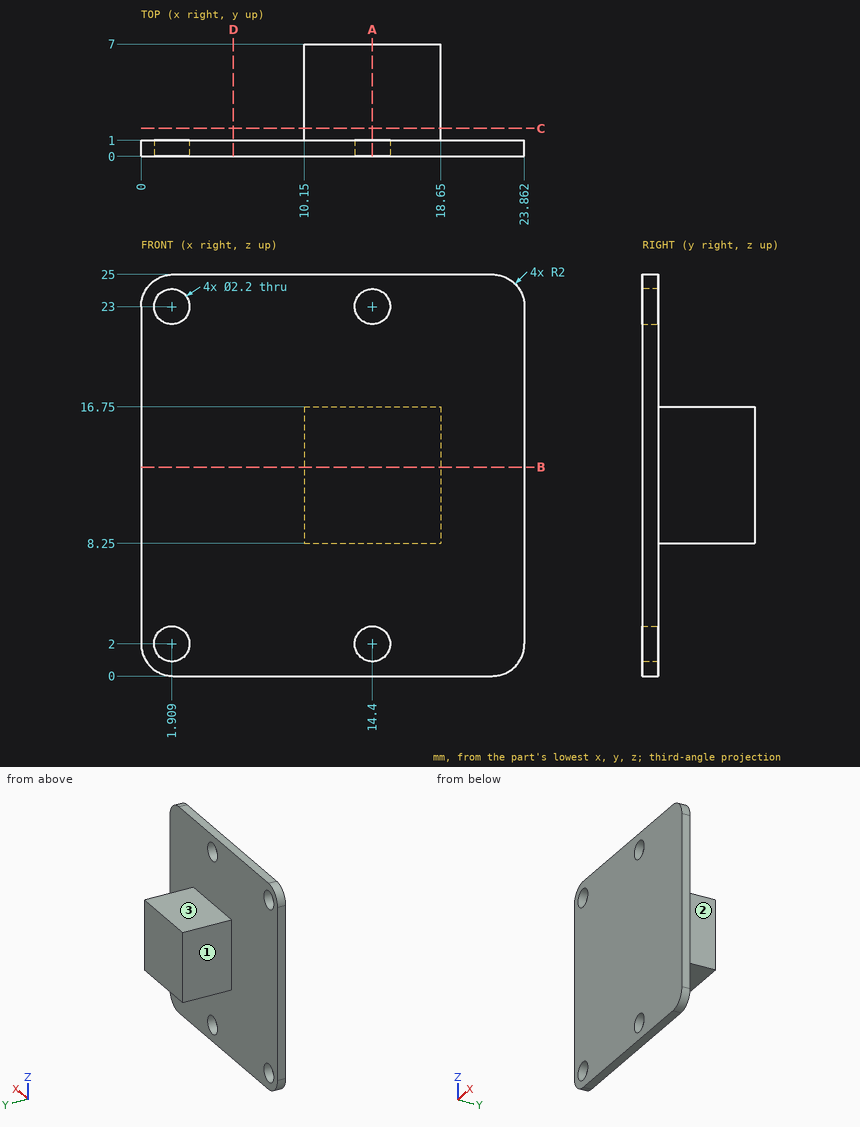
The figure shows three views and two pictorial views of one solid part (mm, origin at its lowest corner). Answer the questions. A direction names the side the tool comes from. Round coordinates to 2 decimals unless told otherwise and drop trailing zeros. Order: outer loops, then holes, each group sorted by start corner. A loop starts at its lowest first (then second) coordinate and runs counter-clockwise, first axis right, second up. Notation, with made-up numbers: M -6.75,85 L 25.25,85 A14 ccw 25.25,103 Z; hole C 40,2.5 d1. An arc over 180 degrees is marked long. Answer in a Markdown table with one row per item. Add a question column.
1) Which of the six approach directions +Z, -Z, +X, -X, +Y, -Y give full straight-line access (tool end or side, diameter ignored) to the marked faces 1, 2 and 3?
2) The part is cut by section B-B on z = 13. Determine the outline of the cut face in (x, y).
3) Flat-ended cylindrical pins translate along their axes: pin 1 Ø2 at (y, z) = (5.5, 18) entering from +X; pin 2 Ø3 at (x, z) = (1.91, 2) entering from +Y; pin 3 Ø3 at (y, z) = (4, 10.5) entering from -X. Find the tip coordinate at first contact, or state that the pin passes through.
4) The part is cut by section D-D on x = 5.75. Determine the outline of the cut face in (y, z).
5) Consider line 1 along X through (y, z) = (0.5, 23); line 2 along Z through (x, y) = (13.25, 1.25); line 3 along Y through (x, z) = (7.5, 22). Determine where each line is inside the solid, lowest interval first. Write a range as from..to.
6) The part is cut by section C-C on y = 1.75. Determine the outline of the cut face in (x, z).
7) The part is cut by section A-A on x = 14.4. Determine the outline of the cut face in (y, z).
Findings below:
| question | item | result |
|---|---|---|
| 1 | face 1 | +Z, -Z, -X, +Y |
| 1 | face 2 | +Z, -Z, +X, +Y |
| 1 | face 3 | +Z, +X, -X, +Y |
| 2 | outline | M 0,0 L 23.86,0 L 23.86,1 L 18.65,1 L 18.65,7 L 10.15,7 L 10.15,1 L 0,1 Z |
| 3 | pin 1 | passes through |
| 3 | pin 2 | stops at y = 1 |
| 3 | pin 3 | stops at x = 10.15 |
| 4 | outline | M 0,0 L 1,0 L 1,25 L 0,25 Z |
| 5 | line 1 | x = 0..0.81, 3.01..13.3, 15.5..23.86 |
| 5 | line 2 | z = 8.25..16.75 |
| 5 | line 3 | y = 0..1 |
| 6 | outline | M 10.15,8.25 L 18.65,8.25 L 18.65,16.75 L 10.15,16.75 Z |
| 7 | outline | M 0,0 L 1,0 L 1,0.9 L 0,0.9 Z; M 0,3.1 L 1,3.1 L 1,8.25 L 7,8.25 L 7,16.75 L 1,16.75 L 1,21.9 L 0,21.9 Z; M 0,24.1 L 1,24.1 L 1,25 L 0,25 Z |
